Build history of the part. All positions in model axes, mm. Face numbers are marked on the shaded views. Coordinates: 2 decimals unless noted, no trailing zeros. Order: outer loops, then holes, each group sorted by start corner. A loop starts at its lowest first (then second) coordinate and runs counter-clockwise, first axis right, second up. Notation, with made-up numbers: M -15,-19.75 L 42,-19.75 A27 ccw 42,5.25 Z; hole C 81.25,67 d4. An arc over 180 degrees is marked long. Use a Markdown table: item, result. Add a question column.
from build123d import *

# Parameters (mm, degrees)
EXTRUDE_1_DEPTH    = 6.35
HOLE_WIZARD_M5_1_D = 5.5


with BuildPart() as part:
    # 스케치1 → 보스-돌출1 (new body)
    with BuildSketch(Plane(origin=(0, 0, 0), x_dir=(1, 0, 0), z_dir=(0, 1, 0))):
        with BuildLine():
            Line((-18.83, 25), (18.83, 25))
            ThreePointArc((18.83, 25), (23.19284884, 23.19284884), (25, 18.83))
            Line((25, 18.83), (25, -18.83))
            ThreePointArc((25, -18.83), (23.19284884, -23.19284884), (18.83, -25))
            Line((18.83, -25), (-18.83, -25))
            ThreePointArc((-18.83, -25), (-23.19284884, -23.19284884), (-25, -18.83))
            Line((-25, -18.83), (-25, 18.83))
            ThreePointArc((-25, 18.83), (-23.19284884, 23.19284884), (-18.83, 25))
        make_face()
    extrude(amount=-EXTRUDE_1_DEPTH)

    # M5 여유 구멍1 (through all)
    with Locations(Plane(origin=(0, 0, 0), x_dir=(1, 0, 0), z_dir=(0, 1, 0))):
        with Locations((0, 10), (10, 0), (0, -10), (-10, 0), (0, 0)):
            Hole(HOLE_WIZARD_M5_1_D / 2)


solid = part.part
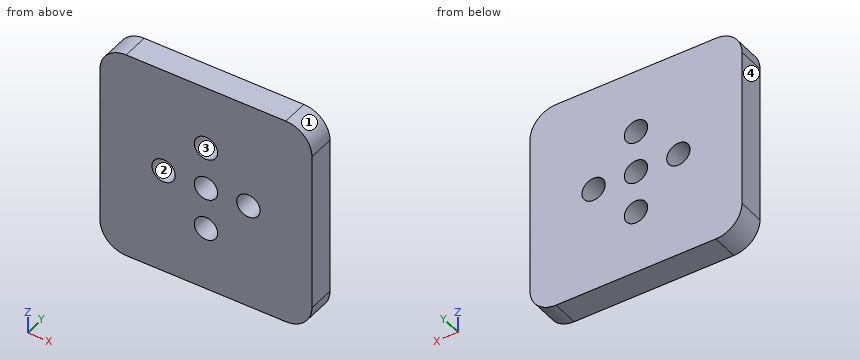
(1) Slice it at A-A on z = -10. Give the cut face in (x, y), and give its area (3 significant figures).
(2) Slice it at B-B on y = -1.5. Give the cut face in (x, z), and give its area (3 significant figures).
(3) Mould opens along Z. For the marked faces 1, 2, 3 and 4 say: released by +Z, released by -Z, zero draft, split by the parting line, or undercut.
(4) Drop a flat-ended pin along its axis: P1, Ø5, axis at x = 0, z = 0, coming from the -Y side. Give the stop position or say it passes through.
(5) Slice it at D-D on x = 0. Give the cut face in (y, z).
(6) Slice it at C-C on x = -10. Give the cut face in (y, z).
(7) Drill centre lines: line 1 along Z through (x, y) = (0, -2); line 2 along Z through (x, y) = (10, -2.5). Where is each one in solid material? Low to high. Write a range as from..to.
Solutions:
| question | item | result |
|---|---|---|
| 1 | outline | M -25,-6.35 L -2.75,-6.35 L -2.75,0 L -25,0 Z; M 2.75,-6.35 L 25,-6.35 L 25,0 L 2.75,0 Z |
| 1 | area | 283 mm² |
| 2 | outline | M -25,-18.83 A6.17 ccw -18.83,-25 L 18.83,-25 A6.17 ccw 25,-18.83 L 25,18.83 A6.17 ccw 18.83,25 L -18.83,25 A6.17 ccw -25,18.83 Z; hole C -10,0 d5.5; hole C 0,-10 d5.5; hole C 0,0 d5.5; hole C 0,10 d5.5; hole C 10,0 d5.5 |
| 2 | area | 2,350 mm² |
| 3 | face 1 | released by +Z |
| 3 | face 2 | undercut |
| 3 | face 3 | undercut |
| 3 | face 4 | zero draft |
| 4 | P1 | through |
| 5 | outline | M -6.35,-25 L 0,-25 L 0,-12.75 L -6.35,-12.75 Z; M -6.35,-7.25 L 0,-7.25 L 0,-2.75 L -6.35,-2.75 Z; M -6.35,2.75 L 0,2.75 L 0,7.25 L -6.35,7.25 Z; M -6.35,12.75 L 0,12.75 L 0,25 L -6.35,25 Z |
| 6 | outline | M -6.35,-25 L 0,-25 L 0,-2.75 L -6.35,-2.75 Z; M -6.35,2.75 L 0,2.75 L 0,25 L -6.35,25 Z |
| 7 | line 1 | -25..-12.75, -7.25..-2.75, 2.75..7.25, 12.75..25 |
| 7 | line 2 | -25..-2.75, 2.75..25 |
